from build123d import *

# Parameters (mm, degrees)
SKETCH_1_R      = 2.95
SKETCH_1_R_2    = 3.4
EXTRUDE_1_DEPTH = 205


with BuildPart() as part:
    # 草图1 → 凸台-拉伸1 (new body, symmetric)
    with BuildSketch(Plane.XY.offset(50)):
        with BuildLine():
            Line((-1518.245004392, 3588.004280474), (-1518.245004392, 3582.975600817))
            Line((-1518.245004392, 3582.975600817), (-1522.916324736, 3578.304280474))
            Line((-1522.916324736, 3578.304280474), (-1533.673684048, 3578.304280474))
            Line((-1533.673684048, 3578.304280474), (-1538.345004392, 3582.975600817))
            Line((-1538.345004392, 3582.975600817), (-1538.345004392, 3588.004280474))
            Line((-1538.345004392, 3588.004280474), (-1534.845004392, 3588.004280474))
            Line((-1534.845004392, 3588.004280474), (-1534.845004392, 3586.304280474))
            Line((-1534.845004392, 3586.304280474), (-1532.445004392, 3586.304280474))
            Line((-1532.445004392, 3586.304280474), (-1532.445004392, 3589.704280474))
            ThreePointArc((-1532.445004392, 3589.704280474), (-1532.503583036, 3589.84570183), (-1532.645004392, 3589.904280474))
            Line((-1532.645004392, 3589.904280474), (-1533.345004392, 3589.904280474))
            Line((-1533.345004392, 3589.904280474), (-1533.345004392, 3590.604280474))
            ThreePointArc((-1533.345004392, 3590.604280474), (-1533.403583036, 3590.74570183), (-1533.545004392, 3590.804280474))
            Line((-1533.545004392, 3590.804280474), (-1543.795004392, 3590.804280474))
            ThreePointArc((-1543.795004392, 3590.804280474), (-1546.976984907, 3589.486260989), (-1548.295004392, 3586.304280474))
            Line((-1548.295004392, 3586.304280474), (-1548.295004392, 3576.054280474))
            ThreePointArc((-1548.295004392, 3576.054280474), (-1548.236425748, 3575.912859117), (-1548.095004392, 3575.854280474))
            Line((-1548.095004392, 3575.854280474), (-1547.395004392, 3575.854280474))
            Line((-1547.395004392, 3575.854280474), (-1547.395004392, 3575.154280474))
            ThreePointArc((-1547.395004392, 3575.154280474), (-1547.336425748, 3575.012859117), (-1547.195004392, 3574.954280474))
            Line((-1547.195004392, 3574.954280474), (-1543.795004392, 3574.954280474))
            Line((-1543.795004392, 3574.954280474), (-1543.795004392, 3577.354280474))
            Line((-1543.795004392, 3577.354280474), (-1545.495004392, 3577.354280474))
            Line((-1545.495004392, 3577.354280474), (-1545.495004392, 3580.854280474))
            Line((-1545.495004392, 3580.854280474), (-1540.466324736, 3580.854280474))
            Line((-1540.466324736, 3580.854280474), (-1535.795004392, 3576.18296013))
            Line((-1535.795004392, 3576.18296013), (-1535.795004392, 3565.425600817))
            Line((-1535.795004392, 3565.425600817), (-1540.466324736, 3560.754280474))
            Line((-1540.466324736, 3560.754280474), (-1545.495004392, 3560.754280474))
            Line((-1545.495004392, 3560.754280474), (-1545.495004392, 3564.254280474))
            Line((-1545.495004392, 3564.254280474), (-1543.795004392, 3564.254280474))
            Line((-1543.795004392, 3564.254280474), (-1543.795004392, 3566.654280474))
            Line((-1543.795004392, 3566.654280474), (-1547.195004392, 3566.654280474))
            ThreePointArc((-1547.195004392, 3566.654280474), (-1547.336425748, 3566.59570183), (-1547.395004392, 3566.454280474))
            Line((-1547.395004392, 3566.454280474), (-1547.395004392, 3565.754280474))
            Line((-1547.395004392, 3565.754280474), (-1548.095004392, 3565.754280474))
            ThreePointArc((-1548.095004392, 3565.754280474), (-1548.236425748, 3565.69570183), (-1548.295004392, 3565.554280474))
            Line((-1548.295004392, 3565.554280474), (-1548.295004392, 3555.304280474))
            ThreePointArc((-1548.295004392, 3555.304280474), (-1546.976984907, 3552.122299958), (-1543.795004392, 3550.804280474))
            Line((-1543.795004392, 3550.804280474), (-1533.545004392, 3550.804280474))
            ThreePointArc((-1533.545004392, 3550.804280474), (-1533.403583036, 3550.862859117), (-1533.345004392, 3551.004280474))
            Line((-1533.345004392, 3551.004280474), (-1533.345004392, 3551.704280474))
            Line((-1533.345004392, 3551.704280474), (-1532.645004392, 3551.704280474))
            ThreePointArc((-1532.645004392, 3551.704280474), (-1532.503583036, 3551.762859117), (-1532.445004392, 3551.904280474))
            Line((-1532.445004392, 3551.904280474), (-1532.445004392, 3555.304280474))
            Line((-1532.445004392, 3555.304280474), (-1534.845004392, 3555.304280474))
            Line((-1534.845004392, 3555.304280474), (-1534.845004392, 3553.604280474))
            Line((-1534.845004392, 3553.604280474), (-1538.345004392, 3553.604280474))
            Line((-1538.345004392, 3553.604280474), (-1538.345004392, 3558.63296013))
            Line((-1538.345004392, 3558.63296013), (-1533.673684048, 3563.304280474))
            Line((-1533.673684048, 3563.304280474), (-1522.916324736, 3563.304280474))
            Line((-1522.916324736, 3563.304280474), (-1518.245004392, 3558.63296013))
            Line((-1518.245004392, 3558.63296013), (-1518.245004392, 3553.604280474))
            Line((-1518.245004392, 3553.604280474), (-1521.745004392, 3553.604280474))
            Line((-1521.745004392, 3553.604280474), (-1521.745004392, 3555.304280474))
            Line((-1521.745004392, 3555.304280474), (-1524.145004392, 3555.304280474))
            Line((-1524.145004392, 3555.304280474), (-1524.145004392, 3551.904280474))
            ThreePointArc((-1524.145004392, 3551.904280474), (-1524.086425748, 3551.762859117), (-1523.945004392, 3551.704280474))
            Line((-1523.945004392, 3551.704280474), (-1523.245004392, 3551.704280474))
            Line((-1523.245004392, 3551.704280474), (-1523.245004392, 3551.004280474))
            ThreePointArc((-1523.245004392, 3551.004280474), (-1523.186425748, 3550.862859117), (-1523.045004392, 3550.804280474))
            Line((-1523.045004392, 3550.804280474), (-1512.795004392, 3550.804280474))
            ThreePointArc((-1512.795004392, 3550.804280474), (-1509.613023877, 3552.122299958), (-1508.295004392, 3555.304280474))
            Line((-1508.295004392, 3555.304280474), (-1508.295004392, 3565.554280474))
            ThreePointArc((-1508.295004392, 3565.554280474), (-1508.353583036, 3565.69570183), (-1508.495004392, 3565.754280474))
            Line((-1508.495004392, 3565.754280474), (-1509.195004392, 3565.754280474))
            Line((-1509.195004392, 3565.754280474), (-1509.195004392, 3566.454280474))
            ThreePointArc((-1509.195004392, 3566.454280474), (-1509.253583036, 3566.59570183), (-1509.395004392, 3566.654280474))
            Line((-1509.395004392, 3566.654280474), (-1512.795004392, 3566.654280474))
            Line((-1512.795004392, 3566.654280474), (-1512.795004392, 3564.254280474))
            Line((-1512.795004392, 3564.254280474), (-1511.095004392, 3564.254280474))
            Line((-1511.095004392, 3564.254280474), (-1511.095004392, 3560.754280474))
            Line((-1511.095004392, 3560.754280474), (-1516.123684048, 3560.754280474))
            Line((-1516.123684048, 3560.754280474), (-1520.795004392, 3565.425600817))
            Line((-1520.795004392, 3565.425600817), (-1520.795004392, 3576.18296013))
            Line((-1520.795004392, 3576.18296013), (-1516.123684048, 3580.854280474))
            Line((-1516.123684048, 3580.854280474), (-1511.095004392, 3580.854280474))
            Line((-1511.095004392, 3580.854280474), (-1511.095004392, 3577.354280474))
            Line((-1511.095004392, 3577.354280474), (-1512.795004392, 3577.354280474))
            Line((-1512.795004392, 3577.354280474), (-1512.795004392, 3574.954280474))
            Line((-1512.795004392, 3574.954280474), (-1509.395004392, 3574.954280474))
            ThreePointArc((-1509.395004392, 3574.954280474), (-1509.253583036, 3575.012859117), (-1509.195004392, 3575.154280474))
            Line((-1509.195004392, 3575.154280474), (-1509.195004392, 3575.854280474))
            Line((-1509.195004392, 3575.854280474), (-1508.495004392, 3575.854280474))
            ThreePointArc((-1508.495004392, 3575.854280474), (-1508.353583036, 3575.912859117), (-1508.295004392, 3576.054280474))
            Line((-1508.295004392, 3576.054280474), (-1508.295004392, 3586.304280474))
            ThreePointArc((-1508.295004392, 3586.304280474), (-1509.613023877, 3589.486260989), (-1512.795004392, 3590.804280474))
            Line((-1512.795004392, 3590.804280474), (-1523.045004392, 3590.804280474))
            ThreePointArc((-1523.045004392, 3590.804280474), (-1523.186425748, 3590.74570183), (-1523.245004392, 3590.604280474))
            Line((-1523.245004392, 3590.604280474), (-1523.245004392, 3589.904280474))
            Line((-1523.245004392, 3589.904280474), (-1523.945004392, 3589.904280474))
            ThreePointArc((-1523.945004392, 3589.904280474), (-1524.086425748, 3589.84570183), (-1524.145004392, 3589.704280474))
            Line((-1524.145004392, 3589.704280474), (-1524.145004392, 3586.304280474))
            Line((-1524.145004392, 3586.304280474), (-1521.745004392, 3586.304280474))
            Line((-1521.745004392, 3586.304280474), (-1521.745004392, 3588.004280474))
            Line((-1521.745004392, 3588.004280474), (-1518.245004392, 3588.004280474))
        make_face()
        with Locations((-1513.270004392, 3555.779280474)):
            Circle(SKETCH_1_R, mode=Mode.SUBTRACT)
        with Locations((-1528.295004392, 3570.804280474)):
            Circle(SKETCH_1_R_2, mode=Mode.SUBTRACT)
        with Locations((-1513.270004392, 3585.829280474)):
            Circle(SKETCH_1_R, mode=Mode.SUBTRACT)
        with Locations((-1543.320004392, 3585.829280474)):
            Circle(SKETCH_1_R, mode=Mode.SUBTRACT)
        with Locations((-1543.320004392, 3555.779280474)):
            Circle(SKETCH_1_R, mode=Mode.SUBTRACT)
    extrude(amount=EXTRUDE_1_DEPTH, both=True)


solid = part.part
CAD build for the part. Positions are in the model's coordinates, mm. A direction names the side the tool comes from. Round coordinates to 2 decimals unless told otherwise and drop trailing zeros. Use a Markdown table: item, result. Add a question column.
1. Slice it at A-A on z = 184. Give the number of separate pieces and of enclosed holes in the cut face, then the cut area to 3 significant figures.
2. Pull direction X, two halves, no side cores. Call faces 1 (the face through (-1508.295, 3560, 53)), 2 (the face through (-1539, 3590.804, 53)), 3 (the face through (-1528, 3563.304, 53)): released by +X, released by -X, zero draft, split by the parting line, or undercut.
3. Drill centre lines: probe 1 along X at (y, z) = (3566, 116.5) (3 decimals); probe 2 along X at (y, z) = (3561, 33.5) (3 decimals); probe 3 along Y at (x, z) = (-1521.5, -95). Where is each one in solid material? Low to high.
4. Flat gauge pins, fed straight in: P1, Ø0.6, axis at x = -1533, z = 66, coming from the -Y side; P2, Ø1.7, axis at x = -1510.5, z = 148.5, coming from the -Y side; P3, Ø1.9, axis at y = 3554, z = 121.5, coming from the +X side. Where does each tip first touch, or does it go through?
5. 3-axis set-ups, long thin cutter, end or side, ignore diameter. For faces 4 (the face through (-1528, 3578.304, 53)), 5 (the face through (-1539, 3550.804, 53)): which of +Z, -Z, +X, -X, +Y, -Y reach the whole face in a straight line?
Reply:
| question | item | result |
|---|---|---|
| 1 | separate pieces | 1 |
| 1 | enclosed holes | 5 |
| 1 | area | 677 mm^2 |
| 2 | face 1 | released by +X |
| 2 | face 2 | zero draft |
| 2 | face 3 | undercut |
| 3 | probe 1 | x = -1547.395 to -1543.795, -1535.795 to -1520.795, -1512.795 to -1509.195 |
| 3 | probe 2 | x = -1548.295 to -1545.495, -1540.221 to -1535.978, -1520.612 to -1516.369, -1511.095 to -1508.295 |
| 3 | probe 3 | y = 3550.8 to 3553.6, 3561.89 to 3579.72, 3588 to 3590.8 |
| 4 | P1 | stops at y = 3551.7 |
| 4 | P2 | stops at y = 3551.04 |
| 4 | P3 | stops at x = -1508.31 |
| 5 | face 4 | +Z, -Z |
| 5 | face 5 | +Z, -Z, +X, -X, -Y |
